Check sheet for the modelled part. Datum: model origin and axes. Units: mm. A direction names the side the tool comes from. Give positions to 0.01 mm unless a question says otherwise; leave off trailing zeros. Loops run counter-clockwise (first coordinate to the right, second up) from the corner with the lowest first, then second, coordinate; pieces in that order, holes last.
```python
from build123d import *

# Parameters (mm, degrees)
PAD_DEPTH    = 19
FILLET_R     = 30
FILLET001_R  = 30
POCKET_DEPTH = 6


with BuildPart() as part:
    # Sketch001 → Pad (new body)
    with BuildSketch(Plane.XZ):
        Polygon((-15, -15), (-15, 115), (147.5259872373, 174.1546216491), (297.0614758428, 585), (485, 516.5959713349), (485, -15), align=None)
    extrude(amount=-PAD_DEPTH)

    # Fillet
    fillet_edges = [part.edges().sort_by_distance(p)[0] for p in [
        (-15, 9.5, 115),
        (-15, 9.5, -15),
        (297.061476, 9.5, 585),
        (485, 9.5, 516.595971),
        (485, 9.5, -15),
    ]]
    fillet(fillet_edges, radius=FILLET_R)

    # Fillet001
    fillet001_edges = [part.edges().sort_by_distance(p)[0] for p in [
        (147.525987, 9.5, 174.154622),
    ]]
    fillet(fillet001_edges, radius=FILLET001_R)

    # Sketch002 (on Face1 of Fillet001) → Pocket (cut)
    with BuildSketch(Plane.XZ):
        Polygon((340.287336399, 569.267073407), (152.1762575699, 52.4361319748), (146.5381018451, 54.4882528347), (334.6491806743, 571.319194267), align=None)
    extrude(amount=-POCKET_DEPTH, mode=Mode.SUBTRACT)


solid = part.part
```
(1) Gauge pin test, flat end, axial feed: pin 1 Ø10 at (x, y) = (94.5, 9.5) entering from +Z. Record the tip position at first contact, or that the pin passes through.
(2) Section check A-A on y = 13. Record the boundary of the cut face in (x, z).
(3) Material ranges on line 1 (X direction, y = 3, z = 348); line 2 (Z direction, x = 33, y = 1.5); line 3 (X direction, y = 7.25, z = 194.5), recorded low to high.
(4) Access from +Z, -Z, +X, -X, +Y, -Y to the whole of each face (thin tool, end or side, straight path). Record for faces 1 (the face through (394.276, 9.367, 549.617)), 2 (the face through (244, 6, 313)).
(5) Section check C-C on x = 280. Record the boundary of the cut face in (y, z), plus the area to 3 significant figures.
(6) Section check B-B on z = 346. Record the boundary of the cut face in (x, y), plus the area to 3 significant figures.
(7) Release check for a two-part mould opening along X. For faces 3 (the face through (294, 0, 219)), 4 (the face through (239.28, 2.96, 309.29)), 5 (the face through (479.427, 9.633, 513.007)) record: pulls with the +X half, pulls with the -X half, needs draft (parallel to the pull), parting line crosses it, or undercut.
Computed values:
1. pin 1: stops at z = 156.67
2. outline: (-15, 15) arc R30 ccw to (15, -15) - (455, -15) arc R30 ccw to (485, 15) - (485, 495.59) arc R30 ccw to (465.26, 523.78) - (325.25, 574.74) arc R30 ccw to (286.8, 556.81) - (152.31, 187.3) arc R30 cw to (134.38, 169.37) - (4.74, 122.18) arc R30 ccw to (-15, 93.99) - close
3. line 1: x = 210.8 to 253.37, 259.75 to 485
3. line 2: z = -15 to 132.47
3. line 3: x = 154.93 to 485
4. face 1: +Z, +X, +Y, -Y
4. face 2: -Y
5. outline: (0, -15) - (19, -15) - (19, 538.12) - (0, 538.12) - (0, 421.17) - (6, 421.17) - (6, 403.63) - (0, 403.63) - close
5. area: 10,400 mm2
6. outline: (210.07, 0) - (252.64, 0) - (252.64, 6) - (259.02, 6) - (259.02, 0) - (485, 0) - (485, 19) - (210.07, 19) - close
6. area: 5,190 mm2
7. face 3: needs draft
7. face 4: undercut
7. face 5: pulls with the +X half
